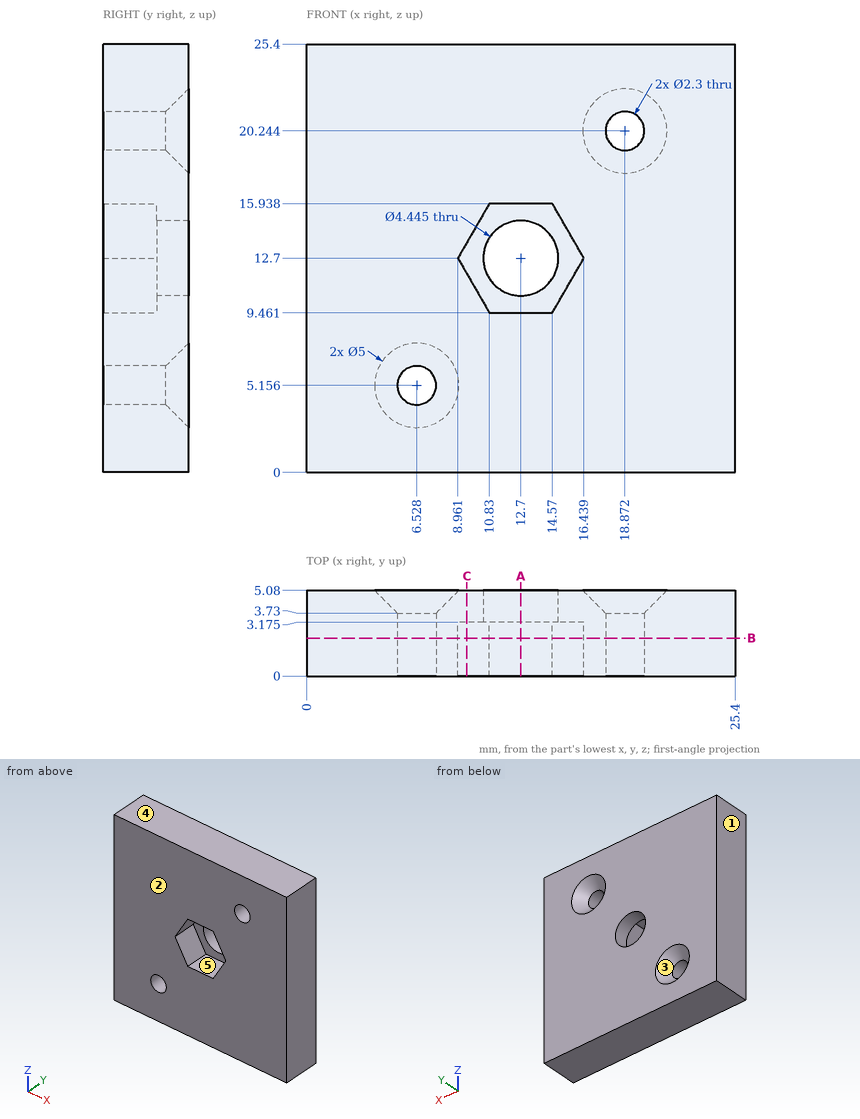
Check sheet for the drawn part. Datum: minimum x, y, z corner. Units: mm. A direction names the side the tool comes from. Coordinates: 2 decimals unless noted, no trailing zeros. Order: outer loops, then holes, each group sorted by start corner. A loop starts at its lowest first (then second) coordinate and runs counter-clockwise, first axis right, second up. Notation, with made-up numbers: (29, 46.25) -> (69, 46.25) arc R6 ccw to (69, 56.25) -> close; hole circle Ø10 at (-6.75, 80.5). An arc over 180 degrees is marked (long way). Use a Markdown table: item, result. Add a question column.
1. Cross-section at B-B (y = 2.25). Enter the section's corners in (x, z).
2. Go/stop test with flat-tipped pins: pin 1 Ø3.5 at (x, z) = (6.53, 5.16) entering from +Y (1 decimal); pin 2 Ø5 at (x, z) = (12.7, 12.7) entering from -Y (1 decimal). Record where each tip stops, or that it passes through.
3. Set-up check for the marked faces 4 and 5: record each of +Z, -Z, +X, -X, +Y, -Y from which the full face is reachable in a straight line by a thin tool's end or side.
4. Cross-section at C-C (x = 9.5). Enter the section's corners in (y, z) (1 decimal).
5. Cross-section at A-A (x = 12.7). Enter the section's corners in (y, z) (1 decimal).
6. Material ranges on L1, parallel to X at y = 1.7, z = 14; L2, parallel to X at y = 2.6, z = 5.75 (1 decimal); L3, parallel to Z at x = 15, y = 2.25 (1 decimal), recorded low to high.
7. Mould release check, pull along X, two halves, no side actions. Record for the marked faces 1, 2 and 3: pulls with the +X half, pulls with the -X half, needs draft (parallel to the pull), parting line crosses it, or undercut.
Filled sheet:
| question | item | result |
|---|---|---|
| 1 | outline | (0, 0) -> (25.4, 0) -> (25.4, 25.4) -> (0, 25.4) -> close; hole circle Ø2.3 at (6.53, 5.16); hole (8.96, 12.7) -> (10.83, 9.46) -> (14.57, 9.46) -> (16.44, 12.7) -> (14.57, 15.94) -> (10.83, 15.94) -> close; hole circle Ø2.3 at (18.87, 20.24) |
| 2 | pin 1 | y = 4.3 |
| 2 | pin 2 | y = 3.2 |
| 3 | face 4 | +Z, +X, -X, +Y, -Y |
| 3 | face 5 | -Y |
| 4 | outline | (0, 0) -> (5.1, 0) -> (5.1, 25.4) -> (0, 25.4) -> (0, 13.6) -> (3.2, 13.6) -> (3.2, 11.8) -> (0, 11.8) -> close |
| 5 | outline | (0, 0) -> (5.1, 0) -> (5.1, 10.5) -> (3.2, 10.5) -> (3.2, 9.5) -> (0, 9.5) -> close; (0, 15.9) -> (3.2, 15.9) -> (3.2, 14.9) -> (5.1, 14.9) -> (5.1, 25.4) -> (0, 25.4) -> close |
| 6 | L1 | 0 to 9.71, 15.69 to 25.4 |
| 6 | L2 | 0 to 5.5, 7.5 to 25.4 |
| 6 | L3 | 0 to 10.2, 15.2 to 25.4 |
| 7 | face 1 | pulls with the -X half |
| 7 | face 2 | needs draft |
| 7 | face 3 | undercut |
